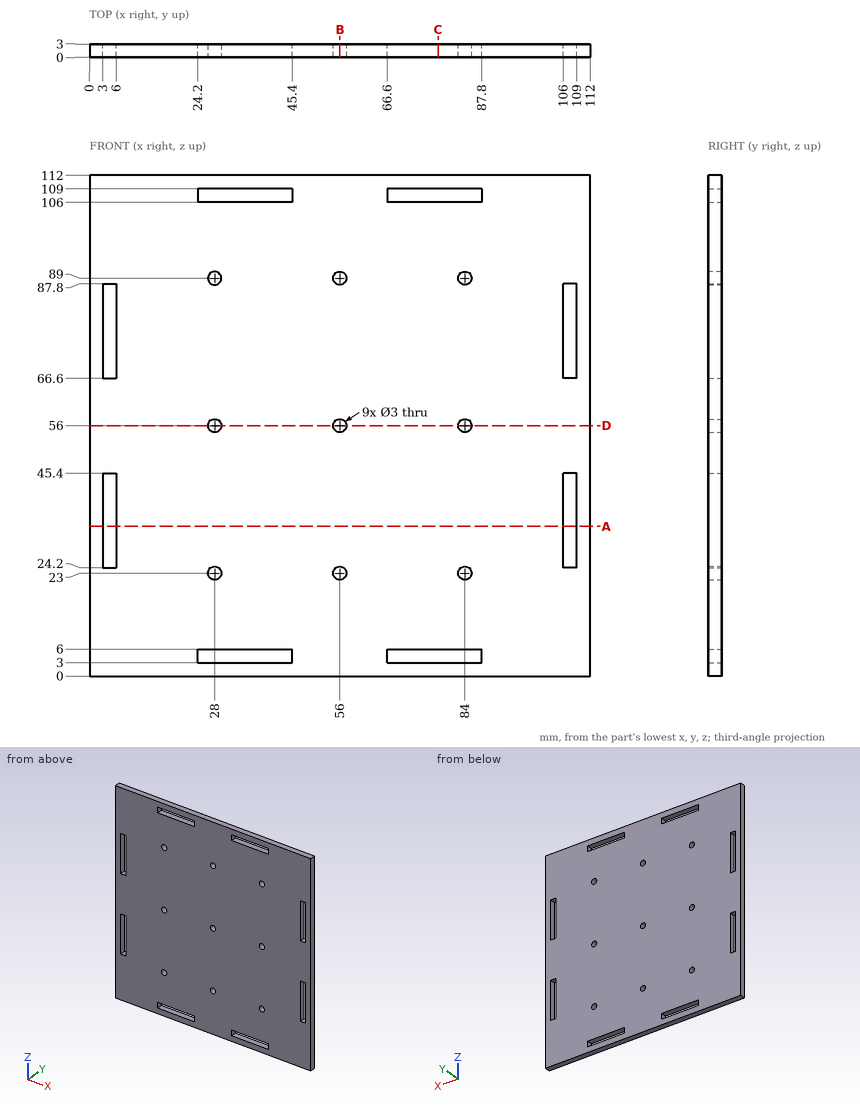
Drawing for the job (mm, zero at the part's lowest x, y, z). Coordinates: 2 decimals unless noted, no trailing zeros. Order: outer loops, then holes, each group sorted by start corner. A loop starts at its lowest first (then second) coordinate and runs counter-clockwise, first axis right, second up. Notation, with made-up numbers: (-27.5, 48) -> (26.5, 48) arc R26 ccw to (26.5, 86) -> close; hole circle Ø10 at (-33, 41). An arc over 180 degrees is marked (long way). Return JSON: item names as keys, results as strings.
Item 1: Slice it at D-D (z = 56). Write the cut outline in (x, y).
Model answer:
{"outline": "(0, 0) -> (26.5, 0) -> (26.5, 3) -> (0, 3) -> close; (29.5, 0) -> (54.5, 0) -> (54.5, 3) -> (29.5, 3) -> close; (57.5, 0) -> (82.5, 0) -> (82.5, 3) -> (57.5, 3) -> close; (85.5, 0) -> (112, 0) -> (112, 3) -> (85.5, 3) -> close"}
Item 2: Wall check: line 1 along Z through (x, y) = (28, 0.9); line 2 along X through (y, z) = (1.5, 35). Give the ranges that are in metal, low to high. Write a range as from..to.
Model answer:
{"line 1": "z = 0..3, 6..21.5, 24.5..54.5, 57.5..87.5, 90.5..106, 109..112", "line 2": "x = 0..3, 6..106, 109..112"}
Item 3: Slice it at C-C (x = 78). Write the cut outline in (y, z), then the cut area to 3 significant figures.
Model answer:
{"outline": "(0, 0) -> (3, 0) -> (3, 3) -> (0, 3) -> close; (0, 6) -> (3, 6) -> (3, 106) -> (0, 106) -> close; (0, 109) -> (3, 109) -> (3, 112) -> (0, 112) -> close", "area": "318 mm²"}
Item 4: Slice it at A-A (z = 33.5). Write the cut outline in (x, y).
Model answer:
{"outline": "(0, 0) -> (3, 0) -> (3, 3) -> (0, 3) -> close; (6, 0) -> (106, 0) -> (106, 3) -> (6, 3) -> close; (109, 0) -> (112, 0) -> (112, 3) -> (109, 3) -> close"}
Item 5: Slice it at B-B (x = 56). Write the cut outline in (y, z), then the cut area to 3 significant figures.
Model answer:
{"outline": "(0, 0) -> (3, 0) -> (3, 21.5) -> (0, 21.5) -> close; (0, 24.5) -> (3, 24.5) -> (3, 54.5) -> (0, 54.5) -> close; (0, 57.5) -> (3, 57.5) -> (3, 87.5) -> (0, 87.5) -> close; (0, 90.5) -> (3, 90.5) -> (3, 112) -> (0, 112) -> close", "area": "309 mm²"}
